Part print with two shaded views. Sizes in mm from the minimum x, y, z corner. A direction names the side the tool comes from. Coordinates: 2 decimals unless noted, no trailing zeros. Order: outer loops, then holes, each group sorted by start corner. A loop starts at its lowest first (then second) coordinate and runs counter-clockwise, first axis right, second up. Notation, with made-up numbers: M -32,-24.75 L 6,-24.75 A31 ccw 6,1.25 Z; hole C 73,37.25 d8. An arc over 180 degrees is marked long. Answer in a Markdown table with one row per item. Add a question column.
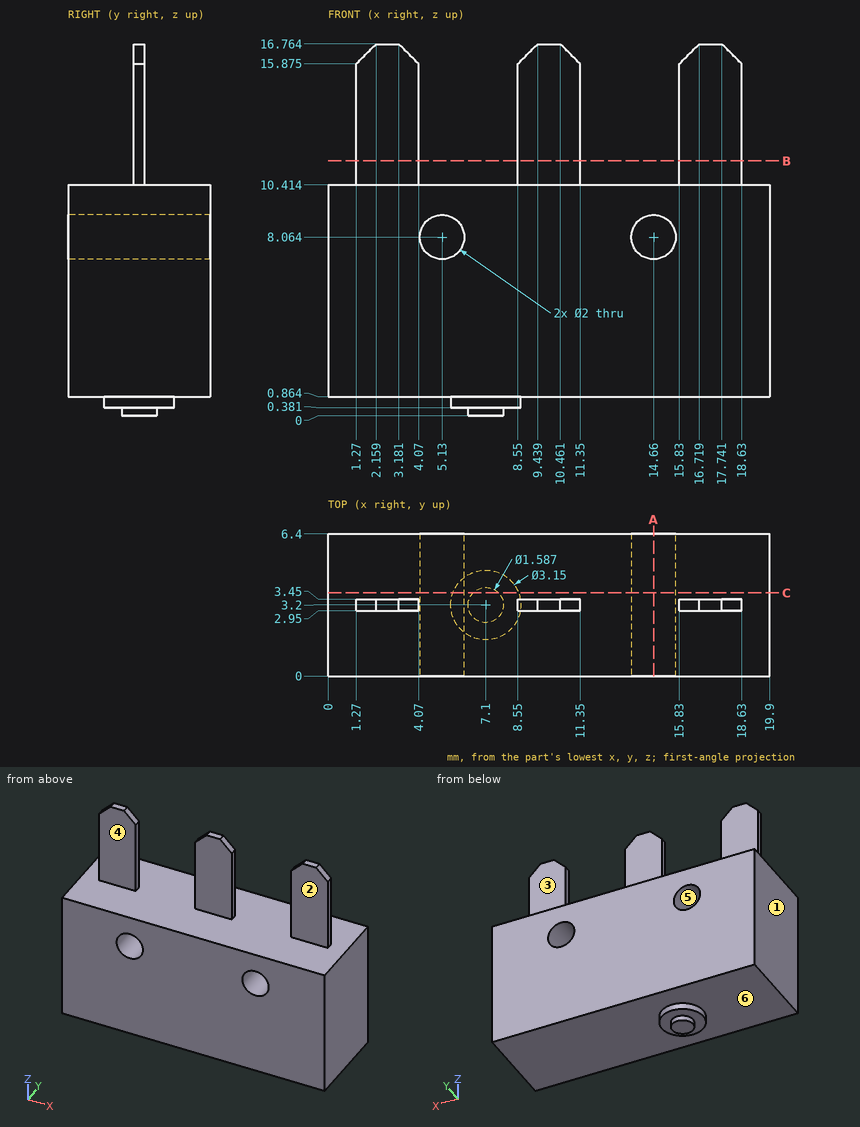
(1) Pull direction Z, two halves, no side cores. Call the marked faces 4, 5 and 6: pulls with the +Z half, pulls with the -Z half, needs draft (parallel to the pull), parting line crosses it, or undercut.
(2) Slice it at A-A (x = 14.66). List the corners of the cut face in (y, z).
(3) 3-axis set-ups, long thin cutter, end or side, ignore diameter. For the marked faces 1, 2 and 3: which of +Z, -Z, +X, -X, +Y, -Y reach the whole face in a straight line?
(4) Wall check: line 1 (X direction, y = 1, z = 8); line 2 (Z direction, x = 5.13, y = 2); line 3 (X direction, y = 2.5, z = 8.75) (1 decimal). Give the ranges that are in metal, low to high.
(5) Drop flat-ended pins along their axis: P1, Ø3, axis at x = 15, y = 2.5, coming from the +Z side (1 decimal); P2, Ø1.4, axis at x = 17.5, z = 12.5, coming from the -Y side; P3, Ø0.8, axis at x = 10, z = 15, coming from the +Y side. Give the stop position or say it passes through.
(6) Slice it at B-B (z = 11.5). List the corners of the cut face in (x, y).
(7) Slice it at C-C (y = 3.75). State how many separate pieces and enclosed holes the cut face has, and give its area (3 significant figures).
Computed:
| question | item | result |
|---|---|---|
| 1 | face 4 | needs draft |
| 1 | face 5 | undercut |
| 1 | face 6 | pulls with the -Z half |
| 2 | outline | M 0,0.86 L 6.4,0.86 L 6.4,7.06 L 0,7.06 Z; M 0,9.06 L 6.4,9.06 L 6.4,10.41 L 0,10.41 Z |
| 3 | face 1 | +Z, -Z, -X, +Y, -Y |
| 3 | face 2 | +Z, +X, -X, -Y |
| 3 | face 3 | +Z, +X, -X, +Y |
| 4 | line 1 | x = 0 to 4.13, 6.13 to 13.66, 15.66 to 19.9 |
| 4 | line 2 | z = 0.86 to 7.06, 9.06 to 10.41 |
| 4 | line 3 | x = 0 to 4.4, 5.9 to 13.9, 15.4 to 19.9 |
| 5 | P1 | stops at z = 16.5 |
| 5 | P2 | stops at y = 2.95 |
| 5 | P3 | stops at y = 3.45 |
| 6 | outline | M 1.27,2.95 L 4.07,2.95 L 4.07,3.45 L 1.27,3.45 Z; M 8.55,2.95 L 11.35,2.95 L 11.35,3.45 L 8.55,3.45 Z; M 15.83,2.95 L 18.63,2.95 L 18.63,3.45 L 15.83,3.45 Z |
| 7 | separate pieces | 1 |
| 7 | enclosed holes | 2 |
| 7 | area | 186 mm^2 |
